Autodesk Inventor part; units mm, degrees
ref_plane "YZ Plane" through (0, 0, 0) normal (1, 0, 0) x (0, 1, 0)
ref_plane "XZ Plane" through (0, 0, 0) normal (0, 1, 0) x (-1, 0, 0)
ref_plane "XY Plane" through (0, 0, 0) normal (0, 0, 1) x (1, 0, 0)
sketch "Sketch1" plane through (0, 0, 0) normal (1, 0, 0) x (0, 1, 0)
  circle A0 centre (0, 0) radius 22.25
  dimension "d0" = 44.5
extrude "Extrusion1" add sketch "Sketch1" along normal blind 135
sketch "Sketch2" plane through (135, 0, 0) normal (1, 0, 0) x (0, 0, -1)
  circle A0 centre (0, 0) radius 4
  line L0 (0, 0) -> (12.3744, 12.3744) construction
  line L1 (0, 0) -> (17.5, 0) construction
  line L2 (0, 0) -> (-12.3744, -12.3744) construction
  line L3 (0, 0) -> (17.5, 0) construction
  circle A1 centre (-12.3744, -12.3744) radius 2
  circle A2 centre (12.3744, 12.3744) radius 2
  circle A3 centre (-12.3744, 12.3744) radius 2
  circle A4 centre (12.3744, -12.3744) radius 2
  circle A5 centre (0, 0) radius 17.5 construction
  dimension "d3" = 8
  dimension "d6" = 17.5
  dimension "d7" = 45
  dimension "d8" = 17.5
  dimension "d9" = 135
  dimension "d10" = 4
  dimension "d11" = 4
extrude "Extrusion2" add sketch "Sketch2" along normal blind 23 contours A0
extrude "Extrusion3" cut sketch "Sketch2" against normal blind 5 contours A1 | A2 | A3 | A4
properties part number "MOOOOT"
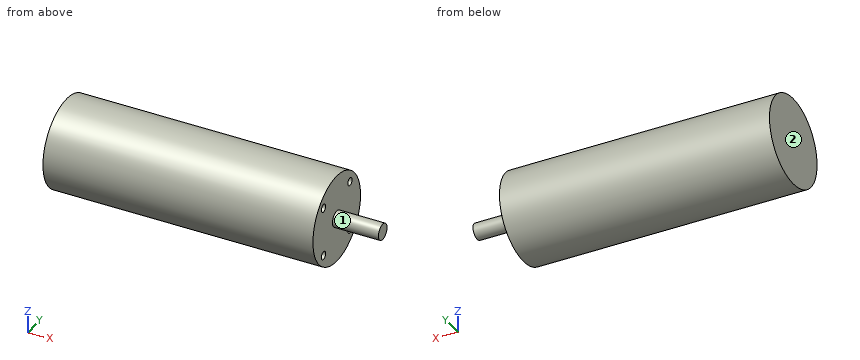
Model file for the job. Use its own axes, mm. Face numbers are marked on the shaded views. A direction names the side the tool comes from. Give positions to 0.01 mm unless a question says otherwise; leave off trailing zeros. Order: outer loops, then holes, each group sorted by start corner. A loop starts at its lowest first (then second) coordinate and runs counter-clockwise, first axis right, second up. Notation, with made-up numbers: (-28, -6) - (16, -6) arc R14 ccw to (16, 15) - close; hole circle Ø4 at (54, -5.5). An arc over 180 degrees is marked (long way). One line per item, written item: value.
Item 1: Slice it at A-A (z = 0). List the corners of the cut face in (x, y).
Response values:
outline: (0, -22.25) - (135, -22.25) - (135, -4) - (158, -4) - (158, 4) - (135, 4) - (135, 22.25) - (0, 22.25) - close
Item 2: Wall check: line 1 (X direction, y = 5.5, z = -10); line 2 (Z direction, x = 105.5, y = -17); line 3 (Z direction, x = 111, y = -1). Give the ranges that are in metal, low to high.
Response values:
line 1: 0 to 135
line 2: -14.35 to 14.35
line 3: -22.23 to 22.23
Item 3: Slice it at D-D (z = 7). List the corners of the cut face in (x, y).
Response values:
outline: (0, -21.12) - (135, -21.12) - (135, 21.12) - (0, 21.12) - close
Item 4: Pin check, flat tips, straight feed: pin 1 Ø4.5 at (y, z) = (-11.5, 11.5) entering from +X; pin 2 Ø4 at (x, y) = (52.5, 6) entering from -Z; pin 3 Ø10 at (x, z) = (47, -16.5) entering from +Y. Stop position of each tip, or through.
Response values:
pin 1: x = 135
pin 2: z = -21.89
pin 3: y = 19.05
Item 5: Slice it at C-C (x = 124.5). List the corners of the cut face in (y, z), then the cut area to 3 significant figures.
Response values:
outline: circle Ø44.5 at (0, 0)
area: 1,560 mm2
Item 6: Tool access for the marked faces 1 and 2: list every direction of +Z, -Z, +X, -X, +Y, -Y with a clear straight run to the whole face (end or side of a thin tool).
Response values:
face 1: +X
face 2: +Z, -Z, -X, +Y, -Y
